Source: CAD feature listing. Evaluate the final solid. Frame: model axes, mm. Give positions to 0.01 mm unless a question says otherwise; leave off trailing zeros. Order: outer loops, then holes, each group sorted by start corner. A loop starts at its lowest first (then second) coordinate and runs counter-clockwise, first axis right, second up.
from build123d import *

# Parameters (mm, degrees)
F0_R     = 12.5
F0_W     = 22.75
F0_H     = 26
F1_DEPTH = 2
F2_DEPTH = 25
F3_R     = 2
F4_D     = 8.2


# Not quite as in the source:
# - a feature names something its author has since deleted; it is built from what else it names


with BuildPart() as f1:
    # F0 (on Top) → F1 (new body)
    with BuildSketch(Plane.XY):
        with BuildLine():
            Line((-22.75, 1.5), (-22.75, 27.5))
            Line((-22.75, 27.5), (0, 27.5))
            Line((0, 27.5), (0, 34.5))
            Line((0, 34.5), (-40, 34.5))
            ThreePointArc((-40, 34.5), (-52.3743686708, 29.3743686708), (-57.5, 17))
            Line((-57.5, 17), (-57.5, -17))
            ThreePointArc((-57.5, -17), (-56.6642107828, -22.3436016868), (-54.2366766871, -27.1767891256))
            Line((-54.2366766871, -27.1767891256), (-50.3051172775, -32.6767891256))
            ThreePointArc((-50.3051172775, -32.6767891256), (-44.0733200493, -38.0618734363), (-36.0684405904, -40))
            Line((-36.0684405904, -40), (0, -40))
            Line((0, -40), (0, -33))
            Line((0, -33), (-22.75, -33))
            Line((-22.75, -33), (-22.75, -7))
            Line((-22.75, -7), (0, -7))
            Line((0, -7), (0, 1.5))
            Line((0, 1.5), (-22.75, 1.5))
        make_face()
        with Locations((-40, -17)):
            Circle(F0_R, mode=Mode.SUBTRACT)
        with Locations((-40, 17)):
            Circle(F0_R, mode=Mode.SUBTRACT)
        with Locations((-11.375, 14.5)):
            Rectangle(F0_W, F0_H)
        with Locations((-11.375, -20)):
            Rectangle(F0_W, F0_H)
        with Locations((-40, 17)):
            Circle(F0_R)
        with Locations((-40, -17)):
            Circle(F0_R)
    extrude(amount=F1_DEPTH)

    # F0 (on Top) → F2 (cut)
    with BuildSketch(Plane.XY):
        with Locations((-11.375, 14.5)):
            Rectangle(F0_W, F0_H)
        with Locations((-11.375, -20)):
            Rectangle(F0_W, F0_H)
    extrude(amount=F2_DEPTH, mode=Mode.SUBTRACT)

    # F3
    f3_edges = [f1.edges().sort_by_distance(p)[0] for p in [
        (-22.75, 1.5, 1),
        (-22.75, 27.5, 1),
        (-22.75, -7, 1),
        (-22.75, -33, 1),
    ]]
    fillet(f3_edges, radius=F3_R)

    # F4 (through all)
    with Locations(Plane(origin=(0, 0, 0), x_dir=(1, 0, 0), z_dir=(0, 0, -1))):
        with Locations((-40, -17), (-40, 17)):
            Hole(F4_D / 2)

    # F5: F1 across plane


with BuildPart() as f1_1:
    add(f1.part)
    add(f1.part.mirror(Plane.YZ))


solid = f1_1.part
(1) Section B-B, the plane z = 1.4. Count the separate pieces of the cut face and the enclosed holes in it, plus the area to 3 significant figures.
(2) Section C-C, the plane y = 14. Return loops of the section in (x, z).
(3) Section A-A, the plane x = -1. Return loops of the section in (y, z), plus the area to 3 significant figures.
(4) Pin query (flat end, axial travel): pin 1 Ø0.6 at (y, z) = (18.5, 1.5) entering from +X; pin 2 Ø1 at (y, z) = (-24, 1) entering from +X. Return the tip coordinate at first contact, or that it passes through.
(5) Section D-D, the plane x = -41.5. Return loops of the section in (y, z).
(6) Draft query along Y for faces 1 (the cylindrical face through (36.746, 19.495, 1.014)), 2 (the flat face through (1, -2, 2)), 3 (the cylindrical face through (-56.687, -22.271, 0.986)), 4 (the cylindrical face through (36.746, -14.505, 1.014)). Return one class per face: +Y half, -Y half, draft (parallel to the pull), parting line (faces both ways), or undercut.
(7) Line query: line 1 along Y through (x, z) = (-12.5, 0.5); line 2 along X through (y, z) = (-17, 1.25); line 3 along Y through (x, z) = (-40, 0.65). Output: solid intervals per line, ascending.
Checks:
1. separate pieces: 1
1. enclosed holes: 6
1. area: 5,620 mm2
2. outline: (-57.5, 0) - (-42.79, 0) - (-42.79, 2) - (-57.5, 2) - close; (-37.21, 0) - (-22.75, 0) - (-22.75, 2) - (-37.21, 2) - close; (22.75, 0) - (37.21, 0) - (37.21, 2) - (22.75, 2) - close; (42.79, 0) - (57.5, 0) - (57.5, 2) - (42.79, 2) - close
3. outline: (-40, 0) - (-33, 0) - (-33, 2) - (-40, 2) - close; (-7, 0) - (1.5, 0) - (1.5, 2) - (-7, 2) - close; (27.5, 0) - (34.5, 0) - (34.5, 2) - (27.5, 2) - close
3. area: 45.0 mm2
4. pin 1: stops at x = 57.46
4. pin 2: stops at x = 56.25
5. outline: (-39.14, 0) - (-20.82, 0) - (-20.82, 2) - (-39.14, 2) - close; (-13.18, 0) - (13.18, 0) - (13.18, 2) - (-13.18, 2) - close; (20.82, 0) - (34.44, 0) - (34.44, 2) - (20.82, 2) - close
6. face 1: undercut
6. face 2: draft
6. face 3: -Y half
6. face 4: undercut
7. line 1: y = -40 to -33, -7 to 1.5, 27.5 to 34.5
7. line 2: x = -57.5 to -44.1, -35.9 to -22.75, 22.75 to 35.9, 44.1 to 57.5
7. line 3: y = -39.55 to -21.1, -12.9 to 12.9, 21.1 to 34.5
